from build123d import *

# Parameters (mm, degrees)
F0_R     = 1.5
F1_DEPTH = 1.4


with BuildPart() as f1:
    # F0 (on Top) → F1 (new body)
    with BuildSketch(Plane.XY):
        with BuildLine():
            Line((-19.255053, 85.041668), (-19.55, 80.977936))
            Line((-19.55, 80.977936), (-23.25, 30))
            Line((-23.25, 30), (-23.25, 0))
            Line((-23.25, 0), (-23.25, -30))
            Line((-23.25, -30), (-19.55, -80.977936))
            Line((-19.55, -80.977936), (-19.255053, -85.041668))
            ThreePointArc((-19.255053, -85.041668), (-18.171235, -87.605254), (-15.75, -88.977936))
            Line((-15.75, -88.977936), (0, -91.977936))
            Line((0, -91.977936), (15.75, -88.977936))
            ThreePointArc((15.75, -88.977936), (18.171235, -87.605254), (19.255053, -85.041668))
            Line((19.255053, -85.041668), (19.55, -80.977936))
            Line((19.55, -80.977936), (23.25, -30))
            Line((23.25, -30), (23.25, 0))
            Line((23.25, 0), (23.25, 30))
            Line((23.25, 30), (19.55, 80.977936))
            Line((19.55, 80.977936), (19.255053, 85.041668))
            ThreePointArc((19.255053, 85.041668), (18.171235, 87.605254), (15.75, 88.977936))
            Line((15.75, 88.977936), (0, 91.977936))
            Line((0, 91.977936), (-15.75, 88.977936))
            ThreePointArc((-15.75, 88.977936), (-18.171235, 87.605254), (-19.255053, 85.041668))
        make_face()
        with Locations((-15.75, -80.977936)):
            Circle(F0_R, mode=Mode.SUBTRACT)
        with Locations((-17.25, -30)):
            Circle(F0_R, mode=Mode.SUBTRACT)
        with Locations((15.75, -80.977936)):
            Circle(F0_R, mode=Mode.SUBTRACT)
        with Locations((17.25, -30)):
            Circle(F0_R, mode=Mode.SUBTRACT)
        with Locations((-17.25, 30)):
            Circle(F0_R, mode=Mode.SUBTRACT)
        with Locations((-15.75, 80.977936)):
            Circle(F0_R, mode=Mode.SUBTRACT)
        with BuildLine():
            Line((-14.35, 74.477936), (-14.35, 75.477936))
            Line((-14.35, 75.477936), (-14.35, 76.477936))
            ThreePointArc((-14.35, 76.477936), (-14.057107, 77.185043), (-13.35, 77.477936))
            ThreePointArc((-13.35, 77.477936), (-12.642893, 77.185043), (-12.35, 76.477936))
            Line((-12.35, 76.477936), (-9.5, 76.477936))
            Line((-9.5, 76.477936), (-6.65, 76.477936))
            ThreePointArc((-6.65, 76.477936), (-6.357107, 77.185043), (-5.65, 77.477936))
            ThreePointArc((-5.65, 77.477936), (-4.942893, 77.185043), (-4.65, 76.477936))
            Line((-4.65, 76.477936), (-4.65, 75.477936))
            Line((-4.65, 75.477936), (-4.65, 74.477936))
            ThreePointArc((-4.65, 74.477936), (-4.942893, 73.77083), (-5.65, 73.477936))
            ThreePointArc((-5.65, 73.477936), (-6.357107, 73.77083), (-6.65, 74.477936))
            Line((-6.65, 74.477936), (-9.5, 74.477936))
            Line((-9.5, 74.477936), (-12.35, 74.477936))
            ThreePointArc((-12.35, 74.477936), (-12.642893, 73.77083), (-13.35, 73.477936))
            ThreePointArc((-13.35, 73.477936), (-14.057107, 73.77083), (-14.35, 74.477936))
        make_face(mode=Mode.SUBTRACT)
        with Locations((17.25, 30)):
            Circle(F0_R, mode=Mode.SUBTRACT)
        with BuildLine():
            ThreePointArc((13.35, 77.477936), (14.057107, 77.185043), (14.35, 76.477936))
            Line((14.35, 76.477936), (14.35, 75.477936))
            Line((14.35, 75.477936), (14.35, 74.477936))
            ThreePointArc((14.35, 74.477936), (14.057107, 73.77083), (13.35, 73.477936))
            ThreePointArc((13.35, 73.477936), (12.642893, 73.77083), (12.35, 74.477936))
            Line((12.35, 74.477936), (9.5, 74.477936))
            Line((9.5, 74.477936), (6.65, 74.477936))
            ThreePointArc((6.65, 74.477936), (6.357107, 73.77083), (5.65, 73.477936))
            ThreePointArc((5.65, 73.477936), (4.942893, 73.77083), (4.65, 74.477936))
            Line((4.65, 74.477936), (4.65, 75.477936))
            Line((4.65, 75.477936), (4.65, 76.477936))
            ThreePointArc((4.65, 76.477936), (4.942893, 77.185043), (5.65, 77.477936))
            ThreePointArc((5.65, 77.477936), (6.357107, 77.185043), (6.65, 76.477936))
            Line((6.65, 76.477936), (9.5, 76.477936))
            Line((9.5, 76.477936), (12.35, 76.477936))
            ThreePointArc((12.35, 76.477936), (12.642893, 77.185043), (13.35, 77.477936))
        make_face(mode=Mode.SUBTRACT)
        with Locations((15.75, 80.977936)):
            Circle(F0_R, mode=Mode.SUBTRACT)
    extrude(amount=F1_DEPTH)


solid = f1.part
Input: part model. Units: mm. Frame: model coordinates. Give positions to 0.01 mm unless a question says otherwise; leave off trailing zeros. Order: outer loops, then holes, each group sorted by start corner. A loop starts at its lowest first (then second) coordinate and runs counter-clockwise, first axis right, second up. Notation, with made-up numbers: (47.25, -10) - (55.25, -10) arc R29 ccw to (55.25, 20) - close; hole circle Ø7 at (-15.75, 82). An arc over 180 degrees is marked (long way). Answer as a JSON object with one key per item and string values. Group by question number.
Q1. Cut plane C-C, the plane y = 64. Output: boundary loops of the cut face in (x, z), then the cut area to 3 significant figures.
Q2. Line query: probe 1 along Y at (x, z) = (-18, 1.25); probe 2 along X at (y, z) = (-80.5, 0.9); probe 3 along Y at (x, z) = (-8, 0.7). Output: solid intervals per line, ascending.
Q3. Cut plane B-B, the plane y = -37.5. Output: boundary loops of the cut face in (x, z), then the cut area to 3 significant figures.
Q4. Cut plane A-A, the plane z = 0.35. Count the separate pieces of the cut face and the enclosed holes in it, then the cut area to 3 significant figures.
Q5. First-contact query: pin 1 Ø1.8 at (x, y) = (-15.75, 80.98) entering from +Z; pin 2 Ø0.7 at (x, z) = (-11, 0.5) entering from -Y; pin 3 Ø0.7 at (x, z) = (11, 1) entering from +Y. Flat tips, straight axial feed; report the tip coordinate or a pass-through.
Q6. Mould query, pull axis Y, two halves, no side actions, for faces 1 (the face through (-18.145, 87.635, 0.69)), 2 (the face through (7.76, -90.5, 0.69)), 3 (the face through (14.56, -81.89, 0.69)). Classes: pulls with the +Y half, pulls with the -Y half, needs draft (parallel to the pull), parting line crosses it, or undercut.
Results:
{
 "1": {"outline": "(-20.78, 0) - (20.78, 0) - (20.78, 1.4) - (-20.78, 1.4) - close", "area": "58.2 mm^2"},
 "2": {"probe 1": "-87.79 to -31.3, -28.7 to 28.7, 31.3 to 87.79", "probe 2": "-19.58 to -17.17, -14.33 to 14.33, 17.17 to 19.58", "probe 3": "-90.45 to 74.48, 76.48 to 90.45"},
 "3": {"outline": "(-22.71, 0) - (22.71, 0) - (22.71, 1.4) - (-22.71, 1.4) - close", "area": "63.6 mm^2"},
 "4": {"separate pieces": "1", "enclosed holes": "10", "area": "7,740 mm^2"},
 "5": {"pin 1": "through", "pin 2": "y = -89.95", "pin 3": "y = 89.95"},
 "6": {"face 1": "pulls with the +Y half", "face 2": "pulls with the -Y half", "face 3": "undercut"}
}
